from build123d import *

# Parameters (mm, degrees)
F0_W     = 318
F0_H     = 350
F1_DEPTH = 5
F2_R     = 10
F4_D     = 8
F5_W     = 60
F5_H     = 30
F6_DEPTH = 850
F7_R     = 5
F8_R     = 6
F9_DEPTH = 5


with BuildPart() as f1:
    # F0 (on Top) → F1 (new body)
    with BuildSketch(Plane.XY):
        Rectangle(F0_W, F0_H)
    extrude(amount=F1_DEPTH)

    # F2
    f2_edges = [f1.edges().sort_by_distance(p)[0] for p in [
        (-159, -175, 2.5),
        (159, -175, 2.5),
        (159, 175, 2.5),
        (-159, 175, 2.5),
    ]]
    fillet(f2_edges, radius=F2_R)

    # F4 (through all)
    with Locations(Plane.XY.offset(5)):
        with Locations((-20, -92), (-20, 8), (-20, 108)):
            Hole(F4_D / 2)

    # F5 (on face) → F6 (join)
    with BuildSketch(Plane(origin=(0, 0, 0), x_dir=(1, 0, 0), z_dir=(0, 0, -1))):
        with Locations((0, -50)):
            Rectangle(F5_W, F5_H)
        with Locations((0, -140)):
            Rectangle(F5_W, F5_H)
    extrude(amount=F6_DEPTH)

    # F7
    f7_edges = [f1.edges().sort_by_distance(p)[0] for p in [
        (-30, 125, -425),
        (-30, 155, -425),
        (30, 125, -425),
        (-30, 65, -425),
        (-30, 35, -425),
        (30, 35, -425),
        (30, 65, -425),
        (30, 155, -425),
    ]]
    fillet(f7_edges, radius=F7_R)

    # F8 (on face) → F9 (join)
    with BuildSketch(Plane(origin=(0, 0, -850), x_dir=(1, 0, 0), z_dir=(0, 0, -1))):
        with BuildLine():
            ThreePointArc((100, 65), (97.071068, 72.071068), (90, 75))
            Line((90, 75), (-90, 75))
            ThreePointArc((-90, 75), (-97.071068, 72.071068), (-100, 65))
            Line((-100, 65), (-100, -165))
            ThreePointArc((-100, -165), (-97.071068, -172.071068), (-90, -175))
            Line((-90, -175), (90, -175))
            ThreePointArc((90, -175), (97.071068, -172.071068), (100, -165))
            Line((100, -165), (100, 65))
        make_face()
        with Locations((-60, -135)):
            Circle(F8_R, mode=Mode.SUBTRACT)
        with Locations((60, -135)):
            Circle(F8_R, mode=Mode.SUBTRACT)
        with Locations((-60, 35)):
            Circle(F8_R, mode=Mode.SUBTRACT)
        with BuildLine():
            Line((30, -40), (30, -60))
            ThreePointArc((30, -60), (28.535534, -63.535534), (25, -65))
            Line((25, -65), (-25, -65))
            ThreePointArc((-25, -65), (-28.535534, -63.535534), (-30, -60))
            Line((-30, -60), (-30, -40))
            ThreePointArc((-30, -40), (-28.535534, -36.464466), (-25, -35))
            Line((-25, -35), (25, -35))
            ThreePointArc((25, -35), (28.535534, -36.464466), (30, -40))
        make_face(mode=Mode.SUBTRACT)
        with Locations((60, 35)):
            Circle(F8_R, mode=Mode.SUBTRACT)
        with BuildLine():
            ThreePointArc((25, -65), (28.535534, -63.535534), (30, -60))
            Line((30, -60), (30, -40))
            ThreePointArc((30, -40), (28.535534, -36.464466), (25, -35))
            Line((25, -35), (-25, -35))
            ThreePointArc((-25, -35), (-28.535534, -36.464466), (-30, -40))
            Line((-30, -40), (-30, -60))
            ThreePointArc((-30, -60), (-28.535534, -63.535534), (-25, -65))
            Line((-25, -65), (25, -65))
        make_face()
    extrude(amount=F9_DEPTH)


solid = f1.part
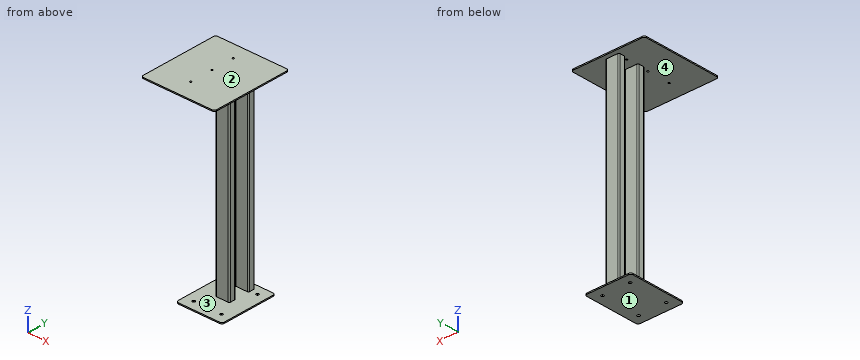
Geometry: final body of the model. Coordinates: model frame, mm. Face numbers are marked on the shaded views. Round coordinates to 2 decimals unless told otherwise and drop trailing zeros. Order: outer loops, then holes, each group sorted by start corner. A loop starts at its lowest first (then second) coordinate and runs counter-clockwise, first axis right, second up.
Q1. Section A-A, the plane x = 43.5. Output: boundary loops of the cut face in (y, z), and give its area (3 significant figures).
Result sheet:
outline: (-175, 0) - (175, 0) - (175, 5) - (-175, 5) - close; (-75, -855) - (175, -855) - (175, -850) - (-75, -850) - close
area: 3,000 mm2
Q2. Mould query, pull axis Z, two halves, no side actions, for the marked faces 1, 2, 3 and 4. Classes: released by +Z, released by -Z, zero draft, split by the parting line, or undercut.
Result sheet:
face 1: released by -Z
face 2: released by +Z
face 3: undercut
face 4: undercut
Q3. Pin query (flat end, axial travel): pin 1 (11 mm diameter, centred on x = -60, y = -35, fed in from -Z); pin 2 (25 mm diameter, centred on x = -11.5, z = -360, fed in from -Y); pin 3 (2.5 mm diameter, centred on x = -31.5, z = -853, fed in from -Y). Return the tip coordinate at first contact, or that it passes through.
Result sheet:
pin 1: stops at z = 0
pin 2: stops at y = 35
pin 3: stops at y = -75
Q4. Section D-D, the plane y = -130.5. Output: boundary loops of the cut face in (x, z).
Result sheet:
outline: (-159, 0) - (159, 0) - (159, 5) - (-159, 5) - close
Q5. Section B-B, the plane y = 89. Output: boundary loops of the cut face in (x, z).
Result sheet:
outline: (-159, 0) - (159, 0) - (159, 5) - (-159, 5) - close; (-100, -855) - (100, -855) - (100, -850) - (-100, -850) - close
Q6. Section C-C, the plane z = -98.5. Output: boundary loops of the cut face in (x, y), and give its area (3 significant figures).
Result sheet:
outline: (-30, 40) arc R5 ccw to (-25, 35) - (25, 35) arc R5 ccw to (30, 40) - (30, 60) arc R5 ccw to (25, 65) - (-25, 65) arc R5 ccw to (-30, 60) - close; (-30, 130) arc R5 ccw to (-25, 125) - (25, 125) arc R5 ccw to (30, 130) - (30, 150) arc R5 ccw to (25, 155) - (-25, 155) arc R5 ccw to (-30, 150) - close
area: 3,560 mm2
Q7. Material intervals for probe 1 along X at (y, z) = (135, -852.7); probe 2 along Y at (x, z) = (-60, -853.9); probe 3 along Z at (x, y) = (71, 103.5), sorted ascending.
Result sheet:
probe 1: x = -100 to -66, -54 to 54, 66 to 100
probe 2: y = -75 to -41, -29 to 129, 141 to 175
probe 3: z = -855 to -850, 0 to 5
